```python
from build123d import *

# Parameters (mm, degrees)
F0_R     = 3
F1_DEPTH = 3


with BuildPart() as f1:
    # F0 (on Top) → F1 (new body)
    with BuildSketch(Plane.XY):
        with BuildLine():
            ThreePointArc((67.24837, -60.331655), (73.009251, -49.555831), (75, -37.5))
            ThreePointArc((75, -37.5), (73.734834, -27.841491), (70.024705, -18.834696))
            ThreePointArc((70.024705, -18.834696), (53.381141, -17.534216), (41.443412, -29.204267))
            ThreePointArc((41.443412, -29.204267), (39.349684, -30.787351), (36.995309, -29.626849))
            ThreePointArc((36.995309, -29.626849), (39.655951, -9.080062), (60.331655, -7.75163))
            ThreePointArc((60.331655, -7.75163), (40.003324, -0.083648), (18.834696, -4.975295))
            ThreePointArc((18.834696, -4.975295), (17.534216, -21.618859), (29.204267, -33.556588))
            ThreePointArc((29.204267, -33.556588), (30.787351, -35.650316), (29.626849, -38.004691))
            ThreePointArc((29.626849, -38.004691), (9.080062, -35.344049), (7.75163, -14.668345))
            ThreePointArc((7.75163, -14.668345), (0.083648, -34.996676), (4.975295, -56.165304))
            ThreePointArc((4.975295, -56.165304), (21.618859, -57.465784), (33.556588, -45.795733))
            ThreePointArc((33.556588, -45.795733), (35.650316, -44.212649), (38.004691, -45.373151))
            ThreePointArc((38.004691, -45.373151), (35.344049, -65.919938), (14.668345, -67.24837))
            ThreePointArc((14.668345, -67.24837), (34.996676, -74.916352), (56.165304, -70.024705))
            ThreePointArc((56.165304, -70.024705), (57.465784, -53.381141), (45.795733, -41.443412))
            ThreePointArc((45.795733, -41.443412), (44.212649, -39.349684), (45.373151, -36.995309))
            ThreePointArc((45.373151, -36.995309), (65.919938, -39.655951), (67.24837, -60.331655))
        make_face()
        with Locations((37.5, -37.5)):
            Circle(F0_R, mode=Mode.SUBTRACT)
    extrude(amount=F1_DEPTH)


solid = f1.part
```
Can you work these out from the model? Positions are in its coordinate system, mm. A direction names the side the tool comes from. Give positions to 0.01 mm unless a question says otherwise; leave off trailing zeros. Write each loop counter-clockwise with the first axis right and the second up, starting at its lowest first coordinate (ties: lowest second). Pieces come first, ordered by that corner, then holes. Notation, with made-up numbers: (-17.5, 40) - (22.5, 40) arc R28 ccw to (22.5, 73) - close; hole circle Ø11 at (64, 13). An arc over 180 degrees is marked (long way). Write item = value, one per line. Start each with the question number.
1. Imagine slicing it at A-A (z = 1.65). Please give me the cut outline in (x, y), and give its area (3 significant figures).
2. On a 3-axis mill with a long thin cutter (end or side, diameter ignored), from which of +Z, -Z, +X, -X, +Y, -Y can I reach the whole of each face in a straight line? I mean faces 1 (the face through (45, -37, 3)), 2 (the face through (44.217, -39.388, 1.479)). Say none if no direction works.
3. Imagine slicing it at D-D (x = 42.5). Please give me the cut outline in (y, z).
4. Thinking about a two-plate mould opening in X: for faces 3 (the face through (0.106, -34.689, 1.479)), 4 (the face through (40.311, -0.106, 1.479)), 5 (the face through (17.453, -21.392, 1.479)), 6 (the face through (65.703, -39.429, 1.479)), which applies, released by +X, released by -X, zero draft, split by the parting line, or undercut?
5. Imagine slicing it at C-C (y = -51). Please give me the cut outline in (x, z), and give its area (3 significant figures).
6. Please list where these lines run through material, in increasing order: line 1 (Y direction, x = 37.5, z = 2.1); line 2 (X direction, y = -53, z = 0.8); line 3 (Y direction, x = 45, z = 0.2).
7. For pin 1 (1 mm diameter, centred on x = 66, z = 0.5, fed in from +Y); pin 2 (5 mm diameter, centred on x = 37.5, y = -37.5, fed in from -Z), each with a flat end and sliding along its axis, tell me the tip position at first contact or that it passes through.
8. Imagine slicing it at B-B (x = 27). Please give me the cut outline in (y, z).
Worked answers:
q1.outline = (4.98, -56.17) arc R20.2 ccw to (33.56, -45.8) arc R2.5 cw to (38, -45.37) arc R16.3 cw to (14.67, -67.25) arc R37.5 ccw to (56.17, -70.02) arc R20.2 ccw to (45.8, -41.44) arc R2.5 cw to (45.37, -37) arc R16.3 cw to (67.25, -60.33) arc R37.5 ccw to (75, -37.5) arc R37.5 ccw to (70.02, -18.83) arc R20.2 ccw to (41.44, -29.2) arc R2.5 cw to (37, -29.63) arc R16.3 cw to (60.33, -7.75) arc R37.5 ccw to (18.83, -4.98) arc R20.2 ccw to (29.2, -33.56) arc R2.5 cw to (29.63, -38) arc R16.3 cw to (7.75, -14.67) arc R37.5 ccw to start; hole circle Ø6 at (37.5, -37.5)
q1.area = 2,650 mm2
q2.face_1 = +Z, +X, -X, +Y, -Y
q2.face_2 = +Z, -Z
q3.outline = (-74.67, 0) - (-26.92, 0) - (-26.92, 3) - (-74.67, 3) - close; (-6.95, 0) - (-0.33, 0) - (-0.33, 3) - (-6.95, 3) - close
q4.face_3 = released by -X
q4.face_4 = split by the parting line
q4.face_5 = undercut
q4.face_6 = undercut
q5.outline = (2.51, 0) - (30.58, 0) - (30.58, 3) - (2.51, 3) - close; (40.21, 0) - (56.42, 0) - (56.42, 3) - (40.21, 3) - close; (70.33, 0) - (72.49, 0) - (72.49, 3) - (70.33, 3) - close
q5.area = 139 mm2
q6.line_1 = -75 to -63.45, -44.79 to -40.5, -34.5 to -30.21, -11.55 to 0
q6.line_2 = 3.35 to 28.77, 40.46 to 57.32, 70.18 to 71.65
q6.line_3 = -74.24 to -40.94, -37.28 to -23.3, -5.74 to -0.76
q7.pin_1 = -17.01
q7.pin_2 = through
q8.outline = (-73.5, 0) - (-70.08, 0) - (-70.08, 3) - (-73.5, 3) - close; (-54.52, 0) - (-39.34, 0) - (-39.34, 3) - (-54.52, 3) - close; (-32.54, 0) - (-1.5, 0) - (-1.5, 3) - (-32.54, 3) - close
